```python
from build123d import *

# Parameters (mm, degrees)
SKETCH_1_R          = 1.525
SKETCH_1_R_2        = 3.75
EXTRUDE_1_DEPTH     = 3
FILLET_1_R          = 1
SKETCH_2_R          = 1.515
CUT_EXTRUDE_1_DEPTH = 10
CUT_EXTRUDE_2_DEPTH = 10
FILLET_2_R          = 1.2
SKETCH_4_W          = 31
SKETCH_4_H          = 9.5
CUT_EXTRUDE_3_DEPTH = 10
SKETCH_5_W          = 4
SKETCH_5_H          = 9.5
EXTRUDE_1_2_DEPTH   = 3
FILLET_3_R          = 1.5


with BuildPart() as part:
    # 草图1 → Extrude 1 (new body)
    with BuildSketch(Plane.XY):
        with BuildLine():
            Line((-20, -40), (20, -40))
            Line((20, -40), (20, -19))
            Line((20, -19), (8.514771251, 4.212917106))
            ThreePointArc((8.514771251, 4.212917106), (0, 9.5), (-8.514771251, 4.212917106))
            Line((-8.514771251, 4.212917106), (-20, -19))
            Line((-20, -19), (-20, -40))
        make_face()
        with Locations((0, 6.5)):
            Circle(SKETCH_1_R, mode=Mode.SUBTRACT)
        with Locations((6.5, 0)):
            Circle(SKETCH_1_R, mode=Mode.SUBTRACT)
        with Locations((0, -6.5)):
            Circle(SKETCH_1_R, mode=Mode.SUBTRACT)
        with Locations((-6.5, 0)):
            Circle(SKETCH_1_R, mode=Mode.SUBTRACT)
        Circle(SKETCH_1_R_2, mode=Mode.SUBTRACT)
    extrude(amount=EXTRUDE_1_DEPTH)

    # 圆角1
    fillet_1_edges = [part.edges().sort_by_distance(p)[0] for p in [
        (20, -40, 1.5),
        (-20, -40, 1.5),
        (-20, -19, 1.5),
        (20, -19, 1.5),
    ]]
    fillet(fillet_1_edges, radius=FILLET_1_R)

    # 草图2 → 切除-拉伸1 (cut)
    with BuildSketch(Plane(origin=(0, 0, 0), x_dir=(-1, 0, 0), z_dir=(0, 0, -1))):
        with Locations((-15, -37)):
            Circle(SKETCH_2_R)
        with Locations((5, -37)):
            Circle(SKETCH_2_R)
    extrude(amount=-CUT_EXTRUDE_1_DEPTH, mode=Mode.SUBTRACT)

    # 草图3 → 切除-拉伸2 (cut)
    with BuildSketch(Plane(origin=(0, 0, 0), x_dir=(-1, 0, 0), z_dir=(0, 0, -1))):
        with BuildLine():
            Line((-7.743606738, -5.50332215), (-14.421459062, -19))
            Line((-14.421459062, -19), (14.421459062, -19))
            Line((14.421459062, -19), (7.743606738, -5.50332215))
            ThreePointArc((7.743606738, -5.50332215), (0, -9.5), (-7.743606738, -5.50332215))
        make_face()
    extrude(amount=-CUT_EXTRUDE_2_DEPTH, mode=Mode.SUBTRACT)

    # 圆角2
    fillet_2_edges = [part.edges().sort_by_distance(p)[0] for p in [
        (7.743606738, -5.50332215, 1.5),
        (-7.743606738, -5.50332215, 1.5),
        (-14.421459062, -19, 1.5),
        (14.421459062, -19, 1.5),
    ]]
    fillet(fillet_2_edges, radius=FILLET_2_R)

    # 草图4 → 切除-拉伸3 (cut)
    with BuildSketch(Plane(origin=(0, 0, 0), x_dir=(-1, 0, 0), z_dir=(0, 0, -1))):
        with Locations((0, -28.25)):
            Rectangle(SKETCH_4_W, SKETCH_4_H)
    extrude(amount=-CUT_EXTRUDE_3_DEPTH, mode=Mode.SUBTRACT)

    # 草图5 → Extrude 1 2 (add)
    with BuildSketch(Plane(origin=(0, 0, 0), x_dir=(-1, 0, 0), z_dir=(0, 0, -1))):
        with Locations((0, -28.25)):
            Rectangle(SKETCH_5_W, SKETCH_5_H)
    extrude(amount=-EXTRUDE_1_2_DEPTH)

    # 圆角3
    fillet_3_edges = [part.edges().sort_by_distance(p)[0] for p in [
        (15.5, -33, 1.5),
        (15.5, -23.5, 1.5),
        (-15.5, -23.5, 1.5),
        (-15.5, -33, 1.5),
        (2, -33, 1.5),
        (2, -23.5, 1.5),
        (-2, -23.5, 1.5),
        (-2, -33, 1.5),
    ]]
    fillet(fillet_3_edges, radius=FILLET_3_R)


solid = part.part
```
The listing builds one solid part. Answer for the finished solid, in the listing's coordinates (mm). A direction names the side the tool comes from. Coordinates: 2 decimals unless noted, no trailing zeros. Loops run counter-clockwise (first coordinate to the right, second up) from the corner with the lowest first, then second, coordinate; pieces in that order, holes last. Notation, with made-up numbers: (-13, -36) - (11, -36) arc R20 cw to (11, -1) - close; hole circle Ø2 at (-21, 49). An arc over 180 degrees is marked (long way). Write item = value, one per line.
1) Which of the six approach directions +Z, -Z, +X, -X, +Y, -Y give full straight-line access (tool end or side, diameter ignored) to faces 1 (the face through (-9, -23.5, 1)), 2 (the face through (19.699, -39.715, 1.521))?
Responses:
face_1 = +Z, -Z
face_2 = +Z, -Z, +X, -Y
2) Each of these flat-tipped pins is pushed along its axis until it touches: P1, Ø4, axis at x = -5, y = -37, coming from the +Z side; P2, Ø1.5, axis at x = -6.5, z = 2, coming from the +Y side; P3, Ø1.5, axis at x = -7, z = 2.5, coming from the +Y side. Where does it stop, or does it pass through?
Responses:
P1 = 3
P2 = 7.56
P3 = 7.15
3) Determine the mould class of faces 3 (the face through (0.1, 9.5, 1.5)), 4 (the face through (0, -20, 0)), 5 (the face through (7.658, -6.474, 1.521)) for opening direction Y: pulls with the +Y half, pulls with the -Y half, needs draft (parallel to the pull), parting line crosses it, or undercut.
Responses:
face_3 = pulls with the +Y half
face_4 = needs draft
face_5 = undercut
4) Section C-C (z = 1.65) is taken. Count the separate pieces of the cut face and the enclosed holes in it, plus the area to 3 significant figures.
Responses:
separate_pieces = 1
enclosed_holes = 10
area = 973 mm^2
5) Section A-A (y = 0) is taken. Determine the outline of the cut face in (x, z) (3 decimals).
Responses:
outline = (-10.599, 0) - (-8.025, 0) - (-8.025, 3) - (-10.599, 3) - close; (-4.975, 0) - (-3.75, 0) - (-3.75, 3) - (-4.975, 3) - close; (3.75, 0) - (4.975, 0) - (4.975, 3) - (3.75, 3) - close; (8.025, 0) - (10.599, 0) - (10.599, 3) - (8.025, 3) - close
6) Find the intervals of material crossed by line 1 along Y through (x, z) = (0, 1.2) (3 decimals); line 2 along Y through (x, z) = (6.5, 1.2) (3 decimals); line 3 along Y through (x, z) = (15, 0.7) (3 decimals), in increasing order.
Responses:
line_1 = -40 to -19, -9.5 to -8.025, -4.975 to -3.75, 3.75 to 4.975, 8.025 to 9.5
line_2 = -40 to -33, -23.5 to -19, -6.928 to -1.525, 1.525 to 6.928
line_3 = -40 to -38.515, -35.485 to -32.618, -23.882 to -8.894
7) Section B-B (x = 7.5) is taken. Determine the outline of the cut face in (y, z), plus the area to 3 significant figures.
Responses:
outline = (-40, 0) - (-33, 0) - (-33, 3) - (-40, 3) - close; (-23.5, 0) - (-19, 0) - (-19, 3) - (-23.5, 3) - close; (-6.46, 0) - (-1.15, 0) - (-1.15, 3) - (-6.46, 3) - close; (1.15, 0) - (5.83, 0) - (5.83, 3) - (1.15, 3) - close
area = 64.5 mm^2
